Part model, mm, in its own coordinate system. Round coordinates to 2 decimals unless told otherwise and drop trailing zeros. Write each loop counter-clockwise with the first axis right and the second up, starting at its lowest first coordinate (ties: lowest second). Pieces come first, ordered by that corner, then holes. Notation, with made-up numbers: M -28,13 L 1,13 A20 cw 1,50 Z; hole C 37,22.5 d1. An arc over 180 degrees is marked long. Use one line per item in the form item = value. Start each with the question number.
Item 1: Probe L1, parallel to Y at x = 38, z = 2.4; L2, parallel to X at y = 28, z = 1.55; L3, parallel to Y at x = 62.5, z = 2.45. List the from-to ranges inside material, lowest first.
Item 2: Cut at B-B, the plane y = 17. Give the cut face in (x, z).
Item 3: Cut at A-A, the plane x = 49.5. Give the cut face in (y, z), then the cut area to 3 significant figures.
Item 4: Flat gauge pin, fed straight in: pin 1 Ø1 at (x, z) = (54.5, 1) entering from -Y. Where does the tip first touch, or does it go through?
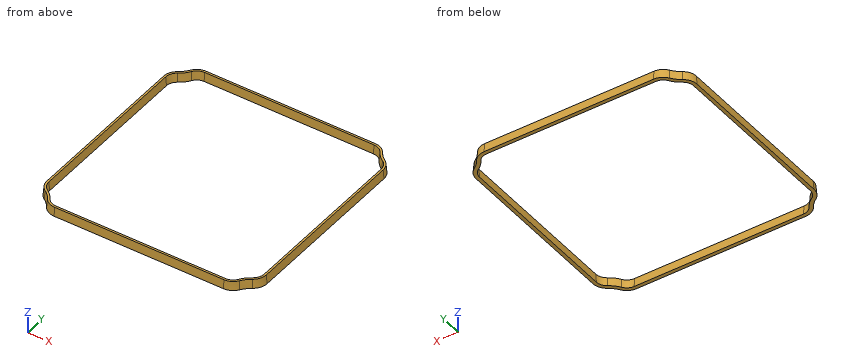
from build123d import *

# Parameters (mm, degrees)
BOSS_EXTRUDE1_DEPTH = 2.5
BOSS_EXTRUDE1_DRAFT = 5


with BuildPart() as part:
    # Sketch1 → Boss-Extrude1 (with draft: the straight prism first)
    with BuildSketch(Plane.XY):
        with BuildLine():
            Line((65.5, 11.25), (65.5, 58.75))
            ThreePointArc((65.5, 58.75), (65.023112089, 60.644117527), (63.706159397, 62.086594179))
            ThreePointArc((63.706159397, 62.086594179), (62.539407406, 63.039407406), (61.586594179, 64.206159397))
            ThreePointArc((61.586594179, 64.206159397), (60.144117527, 65.523112089), (58.25, 66))
            Line((58.25, 66), (10.75, 66))
            ThreePointArc((10.75, 66), (8.855882473, 65.523112089), (7.413405821, 64.206159397))
            ThreePointArc((7.413405821, 64.206159397), (6.460592594, 63.039407406), (5.293840603, 62.086594179))
            ThreePointArc((5.293840603, 62.086594179), (3.976887911, 60.644117527), (3.5, 58.75))
            Line((3.5, 58.75), (3.5, 11.25))
            ThreePointArc((3.5, 11.25), (3.976887911, 9.355882473), (5.293840603, 7.913405821))
            ThreePointArc((5.293840603, 7.913405821), (6.460592594, 6.960592594), (7.413405821, 5.793840603))
            ThreePointArc((7.413405821, 5.793840603), (8.855882473, 4.476887911), (10.75, 4))
            Line((10.75, 4), (58.25, 4))
            ThreePointArc((58.25, 4), (60.144117527, 4.476887911), (61.586594179, 5.793840603))
            ThreePointArc((61.586594179, 5.793840603), (62.539407406, 6.960592594), (63.706159397, 7.913405821))
            ThreePointArc((63.706159397, 7.913405821), (65.023112089, 9.355882473), (65.5, 11.25))
        make_face()
        with BuildLine():
            Line((64.5, 11.25), (64.5, 58.75))
            ThreePointArc((64.5, 58.75), (64.128384354, 60.196235004), (63.105602876, 61.284174304))
            ThreePointArc((63.105602876, 61.284174304), (61.816309207, 62.316309207), (60.784174304, 63.605602876))
            ThreePointArc((60.784174304, 63.605602876), (59.696235004, 64.628384354), (58.25, 65))
            Line((58.25, 65), (10.75, 65))
            ThreePointArc((10.75, 65), (9.303764996, 64.628384354), (8.215825696, 63.605602876))
            ThreePointArc((8.215825696, 63.605602876), (7.183690793, 62.316309207), (5.894397124, 61.284174304))
            ThreePointArc((5.894397124, 61.284174304), (4.871615646, 60.196235004), (4.5, 58.75))
            Line((4.5, 58.75), (4.5, 11.25))
            ThreePointArc((4.5, 11.25), (4.871615646, 9.803764996), (5.894397124, 8.715825696))
            ThreePointArc((5.894397124, 8.715825696), (7.183690793, 7.683690793), (8.215825696, 6.394397124))
            ThreePointArc((8.215825696, 6.394397124), (9.303764996, 5.371615646), (10.75, 5))
            Line((10.75, 5), (58.25, 5))
            ThreePointArc((58.25, 5), (59.696235004, 5.371615646), (60.784174304, 6.394397124))
            ThreePointArc((60.784174304, 6.394397124), (61.816309207, 7.683690793), (63.105602876, 8.715825696))
            ThreePointArc((63.105602876, 8.715825696), (64.128384354, 9.803764996), (64.5, 11.25))
        make_face(mode=Mode.SUBTRACT)
    extrude(amount=BOSS_EXTRUDE1_DEPTH)
    # Boss-Extrude1: the draft: its side faces are tilted about the plane it starts from
    boss_extrude1_sides = [part.faces().sort_by_distance(p)[0] for p in [
        (65.023112089, 9.355882473, 1.25),
        (65.5, 35, 1.25),
        (65.023112089, 60.644117527, 1.25),
        (62.539407406, 63.039407406, 1.25),
        (60.144117527, 65.523112089, 1.25),
        (34.5, 66, 1.25),
        (8.855882473, 65.523112089, 1.25),
        (6.460592594, 63.039407406, 1.25),
        (3.976887911, 60.644117527, 1.25),
        (3.5, 35, 1.25),
        (3.976887911, 9.355882473, 1.25),
        (6.460592594, 6.960592594, 1.25),
        (8.855882473, 4.476887911, 1.25),
        (34.5, 4, 1.25),
        (60.144117527, 4.476887911, 1.25),
        (62.539407406, 6.960592594, 1.25),
        (7.183690793, 7.683690793, 1.25),
        (4.871615646, 9.803764996, 1.25),
        (4.5, 35, 1.25),
        (4.871615646, 60.196235004, 1.25),
        (7.183690793, 62.316309207, 1.25),
        (9.303764996, 64.628384354, 1.25),
        (34.5, 65, 1.25),
        (59.696235004, 64.628384354, 1.25),
        (61.816309207, 62.316309207, 1.25),
        (64.128384354, 60.196235004, 1.25),
        (64.5, 35, 1.25),
        (64.128384354, 9.803764996, 1.25),
        (61.816309207, 7.683690793, 1.25),
        (59.696235004, 5.371615646, 1.25),
        (34.5, 5, 1.25),
        (9.303764996, 5.371615646, 1.25),
    ]]
    draft(boss_extrude1_sides, Plane.XY, BOSS_EXTRUDE1_DRAFT)


solid = part.part
Model answer:
q1.L1 = 4.21 to 4.79, 65.21 to 65.79
q1.L2 = 3.64 to 4.36, 64.64 to 65.36
q1.L3 = 7.22 to 8.01, 61.99 to 62.78
q2.outline = M 3.5,0 L 4.5,0 L 4.28,2.5 L 3.72,2.5 Z; M 64.5,0 L 65.5,0 L 65.28,2.5 L 64.72,2.5 Z
q3.outline = M 4,0 L 5,0 L 4.78,2.5 L 4.22,2.5 Z; M 65,0 L 66,0 L 65.78,2.5 L 65.22,2.5 Z
q3.area = 3.91 mm²
q4.pin_1 = 4.04
